from build123d import *

# Parameters (mm, degrees)
SKETCH1_R               = 279.4
BASE_EXTRUDE_DEPTH      = 25.4
SKETCH5_R               = 12.7
BOSS_EXTRUDE1_DEPTH     = 381
FILLET2_R               = 6.35
CROQUIS1_R              = 88.9
SALIENTE_EXTRUIR1_DEPTH = 12.7


with BuildPart() as part:
    # Sketch1 → Base-Extrude (new body)
    with BuildSketch(Plane.XY):
        Circle(SKETCH1_R)
    extrude(amount=BASE_EXTRUDE_DEPTH)

    # Sketch5 → Boss-Extrude1 (add)
    with BuildSketch(Plane(origin=(0, 0, 0), x_dir=(-1, 0, 0), z_dir=(0, 0, -1))):
        Circle(SKETCH5_R)
    extrude(amount=BOSS_EXTRUDE1_DEPTH)

    # Fillet2
    fillet2_edges = [part.edges().sort_by_distance(p)[0] for p in [
        (-279.4, 0, 0),
        (-279.4, 0, 25.4),
    ]]
    fillet(fillet2_edges, radius=FILLET2_R)

    # Croquis1 → Saliente-Extruir1 (add)
    with BuildSketch(Plane(origin=(0, 0, -381), x_dir=(-1, 0, 0), z_dir=(0, 0, -1))):
        Circle(CROQUIS1_R)
    extrude(amount=SALIENTE_EXTRUIR1_DEPTH)


solid = part.part
The listing builds one solid part. Answer for the finished solid, in the listing's coordinates (mm). A direction names the side the tool comes from. Give positions to 0.01 mm unless a question says otherwise; leave off trailing zeros. Write each loop counter-clockwise with the first axis right and the second up, starting at its lowest first coordinate (ties: lowest second). Pieces come first, ordered by that corner, then holes. Notation, with made-up numbers: (29, 3) - (70, 3) arc R10 cw to (70, 17) - close; hole circle Ø7 at (-27, -7.75). An arc over 180 degrees is marked (long way). One line per question, with ' | ' between items. Start each with the question number.
1. Straight lines are drawn through the part: line 1 (Z direction, x = 118.5, y = -3.5); line 2 (X direction, y = 4, z = -314). For each, find the intervals that lie inside material, in ascending order.
2. Given P1, Ø6, axis at x = -161.5, y = -65, coming from the -Z side; P2, Ø6, axis at y = -5.5, z = -91.5, coming from the +X side; P3, Ø8, axis at x = 6.5, z = -99.5, coming from the -Y side, each flat-ended and moving along its own axis, determine where each tip first touches the part or whether it passes through.
3. Section C-C, the plane z = -207.5 is taken. Determine the outline of the cut face in (x, y).
4. Section A-A, the plane y = 0 is taken. Determine the outline of the cut face in (x, z), then the cut area to 3 significant figures.
5. Determine the mould class of faces 3 (the face through (1, 1, -393.7)), 4 (the face through (-84.795, 26.703, -387.261)), 5 (the face through (1, -19, -381)) for opening direction Z: +Z half, -Z half, draft (parallel to the pull), parting line (faces both ways), or undercut.
6. For faces 1 (the face through (-4, 4, 25.4)), 2 (the face through (2.75, -12.4, -187.83)), determine the directions among +Z, -Z, +X, -X, +Y, -Y from which every point of the face is accessible in a straight line to the end or side of a thin tool.
Result:
1) line 1: z = 0 to 25.4 | line 2: x = -12.05 to 12.05
2) P1: stops at z = 0 | P2: stops at x = 12.45 | P3: stops at y = -12.45
3) outline: circle Ø25.4 at (0, 0)
4) outline: (-279.4, 6.35) arc R6.35 ccw to (-273.05, 0) - (-12.7, 0) - (-12.7, -381) - (-88.9, -381) - (-88.9, -393.7) - (88.9, -393.7) - (88.9, -381) - (12.7, -381) - (12.7, 0) - (273.05, 0) arc R6.35 ccw to (279.4, 6.35) - (279.4, 19.05) arc R6.35 ccw to (273.05, 25.4) - (-273.05, 25.4) arc R6.35 ccw to (-279.4, 19.05) - close | area: 26,100 mm2
5) face 3: -Z half | face 4: draft | face 5: undercut
6) face 1: +Z, +X, -X, +Y, -Y | face 2: none
